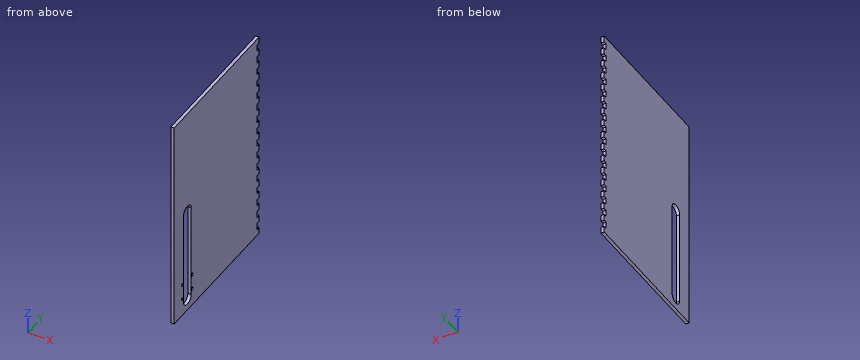
```python
from build123d import *

# Parameters (mm, degrees)
SKETCH1_W           = 431.8
SKETCH1_H           = 285.75
BOSS_EXTRUDE1_DEPTH = 6.35
SKETCH2_W           = 431.8
SKETCH2_H           = 6.35
BOSS_EXTRUDE2_DEPTH = 12.7
CUT_EXTRUDE1_DEPTH  = 20.05
SKETCH5_W           = 51.415141408
SKETCH5_H           = 21.159166417
CUT_EXTRUDE2_DEPTH  = 432.8
SKETCH4_W           = 13.49375
SKETCH4_H           = 6.35
CUT_EXTRUDE3_DEPTH  = 6.35
CUT_EXTRUDE5_DEPTH  = 2.54


with BuildPart() as part:
    # Sketch1 → Boss-Extrude1 (new body)
    with BuildSketch(Plane(origin=(0, 0, 0), x_dir=(0, 0, -1), z_dir=(1, 0, 0))):
        Rectangle(SKETCH1_W, SKETCH1_H)
    extrude(amount=BOSS_EXTRUDE1_DEPTH)

    # Sketch2 → Boss-Extrude2 (add)
    with BuildSketch(Plane(origin=(6.35, 0, 0), x_dir=(0, 0, -1), z_dir=(1, 0, 0))):
        with Locations((0, 139.7)):
            Rectangle(SKETCH2_W, SKETCH2_H)
    extrude(amount=BOSS_EXTRUDE2_DEPTH)

    # Sketch3 → Cut-Extrude1 (cut, through all)
    with BuildSketch(Plane.ZY):
        with BuildLine():
            Line((-190.5, -85.725), (0, -85.725))
            ThreePointArc((0, -85.725), (12.7, -98.425), (0, -111.125))
            Line((0, -111.125), (-190.5, -111.125))
            ThreePointArc((-190.5, -111.125), (-203.2, -98.425), (-190.5, -85.725))
        make_face()
    extrude(amount=-CUT_EXTRUDE1_DEPTH, mode=Mode.SUBTRACT)

    # Sketch5 → Cut-Extrude2 (cut, through all)
    with BuildSketch(Plane(origin=(0, 0, -215.9), x_dir=(-1, 0, 0), z_dir=(0, 0, -1))):
        with Locations((-32.057570704, 147.104583209)):
            Rectangle(SKETCH5_W, SKETCH5_H)
    extrude(amount=-CUT_EXTRUDE2_DEPTH, mode=Mode.SUBTRACT)

    # Sketch4 → Cut-Extrude3 (cut)
    with BuildSketch(Plane.ZY):
        with Locations((-196.453125, 139.7)):
            Rectangle(SKETCH4_W, SKETCH4_H)
        with Locations((-170.259375, 139.7)):
            Rectangle(SKETCH4_W, SKETCH4_H)
        with Locations((-144.065625, 139.7)):
            Rectangle(SKETCH4_W, SKETCH4_H)
        with Locations((-117.871875, 139.7)):
            Rectangle(SKETCH4_W, SKETCH4_H)
        with Locations((-91.678125, 139.7)):
            Rectangle(SKETCH4_W, SKETCH4_H)
        with Locations((-65.484375, 139.7)):
            Rectangle(SKETCH4_W, SKETCH4_H)
        with Locations((-39.290625, 139.7)):
            Rectangle(SKETCH4_W, SKETCH4_H)
        with Locations((-13.096875, 139.7)):
            Rectangle(SKETCH4_W, SKETCH4_H)
        with Locations((13.096875, 139.7)):
            Rectangle(SKETCH4_W, SKETCH4_H)
        with Locations((39.290625, 139.7)):
            Rectangle(SKETCH4_W, SKETCH4_H)
        with Locations((65.484375, 139.7)):
            Rectangle(SKETCH4_W, SKETCH4_H)
        with Locations((91.678125, 139.7)):
            Rectangle(SKETCH4_W, SKETCH4_H)
        with Locations((117.871875, 139.7)):
            Rectangle(SKETCH4_W, SKETCH4_H)
        with Locations((144.065625, 139.7)):
            Rectangle(SKETCH4_W, SKETCH4_H)
        with Locations((170.259375, 139.7)):
            Rectangle(SKETCH4_W, SKETCH4_H)
        with Locations((196.453125, 139.7)):
            Rectangle(SKETCH4_W, SKETCH4_H)
    extrude(amount=-CUT_EXTRUDE3_DEPTH, mode=Mode.SUBTRACT)

    # Sketch6 → Cut-Extrude5 (cut)
    with BuildSketch(Plane(origin=(6.35, 0, 0), x_dir=(0, 0, -1), z_dir=(1, 0, 0))):
        with BuildLine():
            ThreePointArc((152.775, -82.06), (151.84506403, -79.81493597), (149.6, -78.885))
            ThreePointArc((149.6, -78.885), (150.660660172, -79.324339828), (151.1, -80.385))
            Line((151.1, -80.385), (151.1, -84.858325392))
            ThreePointArc((151.1, -84.858325392), (152.324254485, -83.690663209), (152.775, -82.06))
        make_face()
        with BuildLine():
            Line((148.1, -80.385), (148.1, -84.858325392))
            ThreePointArc((148.1, -84.858325392), (149.6, -85.235), (151.1, -84.858325392))
            Line((151.1, -84.858325392), (151.1, -80.385))
            ThreePointArc((151.1, -80.385), (150.660660172, -79.324339828), (149.6, -78.885))
            ThreePointArc((149.6, -78.885), (148.539339828, -79.324339828), (148.1, -80.385))
        make_face()
        with BuildLine():
            ThreePointArc((149.6, -78.885), (146.520608167, -81.286714193), (148.1, -84.858325392))
            Line((148.1, -84.858325392), (148.1, -80.385))
            ThreePointArc((148.1, -80.385), (148.539339828, -79.324339828), (149.6, -78.885))
        make_face()
        with BuildLine():
            Line((179.1, -80.385), (179.1, -84.858325392))
            ThreePointArc((179.1, -84.858325392), (180.6, -85.235), (182.1, -84.858325392))
            Line((182.1, -84.858325392), (182.1, -80.385))
            ThreePointArc((182.1, -80.385), (181.660660172, -79.324339828), (180.6, -78.885))
            ThreePointArc((180.6, -78.885), (179.539339828, -79.324339828), (179.1, -80.385))
        make_face()
        with BuildLine():
            ThreePointArc((180.6, -78.885), (177.520608167, -81.286714193), (179.1, -84.858325392))
            Line((179.1, -84.858325392), (179.1, -80.385))
            ThreePointArc((179.1, -80.385), (179.539339828, -79.324339828), (180.6, -78.885))
        make_face()
        with BuildLine():
            ThreePointArc((183.775, -82.06), (182.84506403, -79.81493597), (180.6, -78.885))
            ThreePointArc((180.6, -78.885), (181.660660172, -79.324339828), (182.1, -80.385))
            Line((182.1, -80.385), (182.1, -84.858325392))
            ThreePointArc((182.1, -84.858325392), (183.324254485, -83.690663209), (183.775, -82.06))
        make_face()
        with BuildLine():
            ThreePointArc((151.1, -116.465), (150.660660172, -117.525660172), (149.6, -117.965))
            ThreePointArc((149.6, -117.965), (151.84506403, -117.03506403), (152.775, -114.79))
            ThreePointArc((152.775, -114.79), (152.324254485, -113.159336791), (151.1, -111.991674608))
            Line((151.1, -111.991674608), (151.1, -116.465))
        make_face()
        with BuildLine():
            Line((148.1, -111.991674608), (148.1, -116.465))
            ThreePointArc((148.1, -116.465), (148.539339828, -117.525660172), (149.6, -117.965))
            ThreePointArc((149.6, -117.965), (150.660660172, -117.525660172), (151.1, -116.465))
            Line((151.1, -116.465), (151.1, -111.991674608))
            ThreePointArc((151.1, -111.991674608), (149.6, -111.615), (148.1, -111.991674608))
        make_face()
        with BuildLine():
            ThreePointArc((149.6, -117.965), (148.539339828, -117.525660172), (148.1, -116.465))
            Line((148.1, -116.465), (148.1, -111.991674608))
            ThreePointArc((148.1, -111.991674608), (146.520608167, -115.563285807), (149.6, -117.965))
        make_face()
        with BuildLine():
            ThreePointArc((180.6, -117.965), (181.660660172, -117.525660172), (182.1, -116.465))
            Line((182.1, -116.465), (182.1, -111.991674608))
            ThreePointArc((182.1, -111.991674608), (180.6, -111.615), (179.1, -111.991674608))
            Line((179.1, -111.991674608), (179.1, -116.465))
            ThreePointArc((179.1, -116.465), (179.539339828, -117.525660172), (180.6, -117.965))
        make_face()
        with BuildLine():
            Line((182.1, -111.991674608), (182.1, -116.465))
            ThreePointArc((182.1, -116.465), (181.660660172, -117.525660172), (180.6, -117.965))
            ThreePointArc((180.6, -117.965), (182.84506403, -117.03506403), (183.775, -114.79))
            ThreePointArc((183.775, -114.79), (183.324254485, -113.159336791), (182.1, -111.991674608))
        make_face()
        with BuildLine():
            ThreePointArc((179.1, -111.991674608), (177.520608167, -115.563285807), (180.6, -117.965))
            ThreePointArc((180.6, -117.965), (179.539339828, -117.525660172), (179.1, -116.465))
            Line((179.1, -116.465), (179.1, -111.991674608))
        make_face()
    extrude(amount=-CUT_EXTRUDE5_DEPTH, mode=Mode.SUBTRACT)


solid = part.part
```
Work out the finished part from the listing and answer in its coordinate system (mm). Coordinates: 2 decimals unless noted, no trailing zeros. Order: outer loops, then holes, each group sorted by start corner. A loop starts at its lowest first (then second) coordinate and runs counter-clockwise, first axis right, second up. Notation, with made-up numbers: (50.5, 29.25) - (77.5, 29.25) arc R25 cw to (77.5, 57.25) - close; hole circle Ø8 at (-7.75, 72.25). An arc over 180 degrees is marked (long way). Answer as a JSON object with one key per item and string values.
1. Find section A-A on z = -63. Determine the outline of the cut face in (x, y) (3 decimals).
Output values:
{"outline": "(0, -142.875) - (6.35, -142.875) - (6.35, -111.125) - (0, -111.125) - close; (0, -85.725) - (6.35, -85.725) - (6.35, 136.525) - (0, 136.525) - close"}
2. Consider line 1 (Y direction, x = 6, z = -35) (3 decimals); line 2 (Y direction, x = 5.5, z = -101) (3 decimals); line 3 (Y direction, x = 1, z = 143) (3 decimals). Determine where each line is inside the solid, lowest interval first.
Output values:
{"line 1": "y = -142.875 to -111.125, -85.725 to 136.525", "line 2": "y = -142.875 to -111.125, -85.725 to 142.875", "line 3": "y = -142.875 to 136.525"}
3. Find section B-B on z = 40. Determine the outline of the cut face in (x, y) (3 decimals).
Output values:
{"outline": "(0, -142.875) - (6.35, -142.875) - (6.35, 136.525) - (0, 136.525) - close"}
4. Each of these flat-tipped pins is pushed along its axis until it touches: P1, Ø1.9, axis at x = 2.5, z = -40.5, coming from the +Y side (3 decimals); P2, Ø3, axis at y = -114, z = -149, coming from the +X side. Where does it stop, or does it pass through?
Output values:
{"P1": "stops at y = 136.525", "P2": "stops at x = 3.81"}
